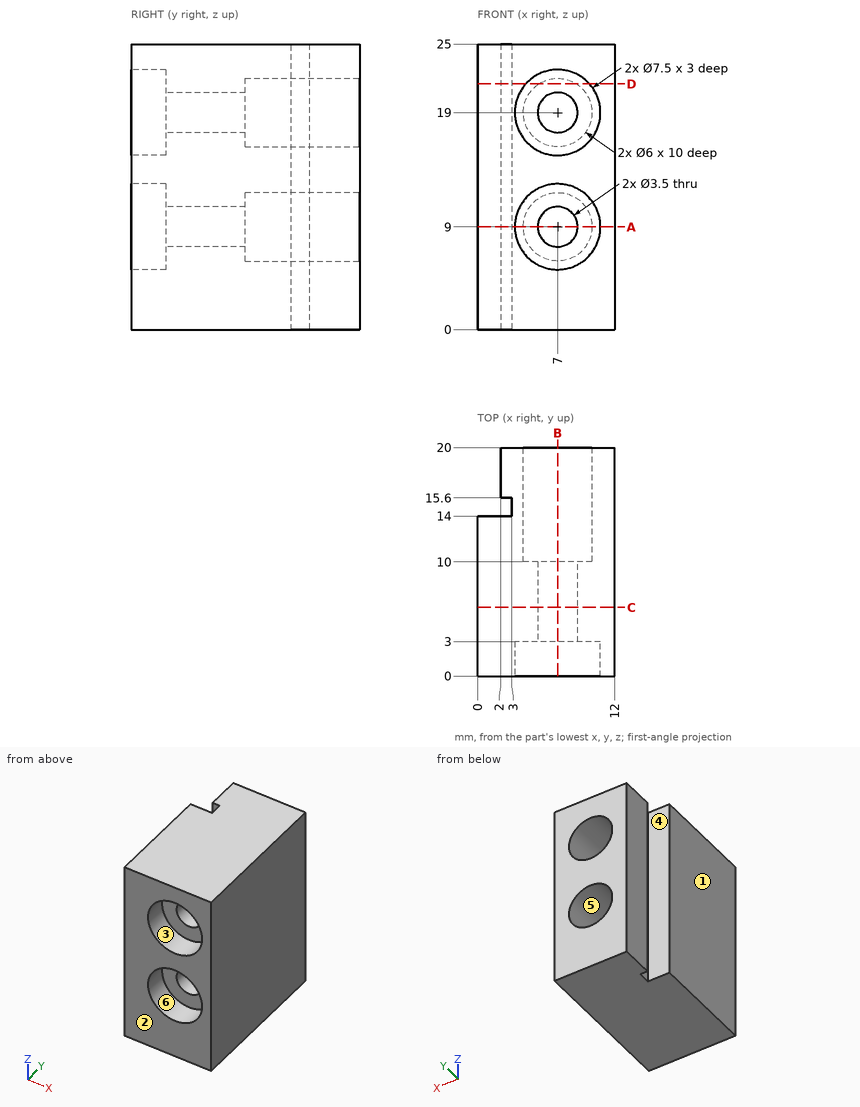
The drawing under review shows one solid part. Ordinate dimensions are in mm from its lowest x, y, z. A direction names the side the tool comes from. Round coordinates to 2 decimals unless told otherwise and drop trailing zeros. Loops run counter-clockwise (first coordinate to the right, second up) from the corner with the lowest first, then second, coordinate; pieces in that order, holes last.
Item 1: For line 1 (Z direction, x = 7, y = 16.25); line 2 (Z direction, x = 7, y = 2.35); line 3 (X direction, y = 17.75, z = 9), list the stretches that pass through material, from the lowest coordinate up.
Determined:
line 1: z = 0 to 6, 12 to 16, 22 to 25
line 2: z = 0 to 5.25, 12.75 to 15.25, 22.75 to 25
line 3: x = 2 to 4, 10 to 12
Item 2: For the marked faces 4, 5 and 6, list the 3-axis set-ups (+Z, -Z, +X, -X, +Y, -Y) from which the entire face can be reached by the end or side of a thin tool; tool diameter is ignored.
Determined:
face 4: +Z, -Z, -X
face 5: +Y
face 6: -Y
Item 3: Mouldability with a two-part tool opening along X and no side actions: class the marked faces 1, 2 and 3 as released by +X, released by -X, zero draft, split by the parting line, or undercut.
Determined:
face 1: released by -X
face 2: zero draft
face 3: undercut
Item 4: Clearance check with flat-ended pins moving along their axes: pin 1 Ø6 at (x, z) = (7.5, 18.5) entering from -Y; pin 2 Ø4.5 at (x, z) = (7, 19) entering from +Y; pin 3 Ø1.8 at (y, z) = (15, 8) entering from -X. State where each tip first meets the part, or that it passes through.
Determined:
pin 1: stops at y = 3
pin 2: stops at y = 10
pin 3: stops at x = 2
Item 5: Take a section at B-B (x = 7). Write out the cut boundary in (y, z), then the cut area to 3 significant figures.
Determined:
outline: (0, 0) - (20, 0) - (20, 6) - (10, 6) - (10, 7.25) - (3, 7.25) - (3, 5.25) - (0, 5.25) - close; (0, 12.75) - (3, 12.75) - (3, 10.75) - (10, 10.75) - (10, 12) - (20, 12) - (20, 16) - (10, 16) - (10, 17.25) - (3, 17.25) - (3, 15.25) - (0, 15.25) - close; (0, 22.75) - (3, 22.75) - (3, 20.75) - (10, 20.75) - (10, 22) - (20, 22) - (20, 25) - (0, 25) - close
area: 286 mm2
Item 6: Take a section at A-A (z = 9). Write out the cut boundary in (x, y), then the cut area to 3 significant figures.
Determined:
outline: (0, 0) - (3.25, 0) - (3.25, 3) - (5.25, 3) - (5.25, 10) - (4, 10) - (4, 20) - (2, 20) - (2, 15.6) - (3, 15.6) - (3, 14) - (0, 14) - close; (8.75, 3) - (10.75, 3) - (10.75, 0) - (12, 0) - (12, 20) - (10, 20) - (10, 10) - (8.75, 10) - close
area: 119 mm2
Item 7: Take a section at D-D (z = 21.5). Write out the cut boundary in (x, y), then the cut area to 3 significant figures.
Determined:
outline: (0, 0) - (4.2, 0) - (4.2, 3) - (9.8, 3) - (9.8, 0) - (12, 0) - (12, 20) - (8.66, 20) - (8.66, 10) - (5.34, 10) - (5.34, 20) - (2, 20) - (2, 15.6) - (3, 15.6) - (3, 14) - (0, 14) - close
area: 176 mm2
Item 8: Take a section at C-C (y = 6). Write out the cut boundary in (x, z).
Determined:
outline: (0, 0) - (12, 0) - (12, 25) - (0, 25) - close; hole circle Ø3.5 at (7, 9); hole circle Ø3.5 at (7, 19)
